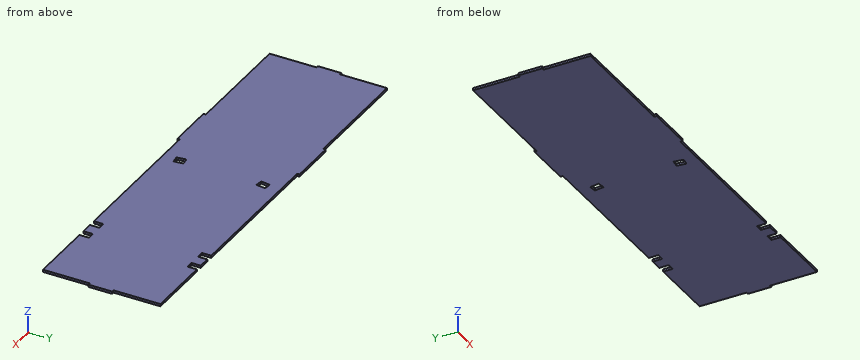
```python
from build123d import *

# Parameters (mm, degrees)
SKETCH_1_W          = 2
SKETCH_1_H          = 20
SKETCH_1_W_2        = 40
SKETCH_1_H_2        = 2
EXTRUDE_1_DEPTH     = 2
CUT_EXTRUDE_1_DEPTH = 10
SKETCH_3_W          = 6
SKETCH_3_H          = 8
CUT_EXTRUDE_2_DEPTH = 2
SKETCH_4_W          = 6
SKETCH_4_H          = 8
CUT_EXTRUDE_3_DEPTH = 2


with BuildPart() as part:
    # 草图1 → 凸台-拉伸1 (new body)
    with BuildSketch(Plane.XY):
        with Locations((1, 50)):
            Rectangle(SKETCH_1_W, SKETCH_1_H)
        Polygon((2, 40), (2, 0), (100, 0), (140, 0), (350, 0), (350, 40), (350, 60), (350, 100), (140, 100), (100, 100), (2, 100), (2, 60), align=None)
        with Locations((120, 101)):
            Rectangle(SKETCH_1_W_2, SKETCH_1_H_2)
        with Locations((120, -1)):
            Rectangle(SKETCH_1_W_2, SKETCH_1_H_2)
        with Locations((351, 50)):
            Rectangle(SKETCH_1_W, SKETCH_1_H)
    extrude(amount=EXTRUDE_1_DEPTH)

    # 草图2 → 切除-拉伸1 (cut)
    with BuildSketch(Plane(origin=(0, 0, 0), x_dir=(-1, 0, 0), z_dir=(0, 0, -1))):
        Polygon((-168.407456688, 81.069541445), (-169.466891791, 88.999080981), (-163.519737138, 89.793657309), (-162.460302035, 81.864117772), align=None)
        Polygon((-162.460302035, 18.135882228), (-168.407456688, 18.930458555), (-169.466891791, 11.000919019), (-163.519737138, 10.206342691), align=None)
    extrude(amount=-CUT_EXTRUDE_1_DEPTH, mode=Mode.SUBTRACT)

    # 草图3 → 切除-拉伸2 (cut)
    with BuildSketch(Plane.XY.offset(2)):
        with Locations((291.061030213, 96)):
            Rectangle(SKETCH_3_W, SKETCH_3_H)
        with Locations((291.061030213, 4)):
            Rectangle(SKETCH_3_W, SKETCH_3_H)
    extrude(amount=-CUT_EXTRUDE_2_DEPTH, mode=Mode.SUBTRACT)

    # 草图4 → 切除-拉伸3 (cut)
    with BuildSketch(Plane.XY.offset(2)):
        with Locations((274.986515691, 4)):
            Rectangle(SKETCH_4_W, SKETCH_4_H)
        with Locations((274.986515691, 96)):
            Rectangle(SKETCH_4_W, SKETCH_4_H)
    extrude(amount=-CUT_EXTRUDE_3_DEPTH, mode=Mode.SUBTRACT)


solid = part.part
```
Here's how the part is built. I have some questions about the finished solid (model axes, mm). Coordinates: 2 decimals unless noted, no trailing zeros. Order: outer loops, then holes, each group sorted by start corner. A loop starts at its lowest first (then second) coordinate and runs counter-clockwise, first axis right, second up. Notation, with made-up numbers: M 9.5,43 L 19.5,43 A28 cw 19.5,67 Z; hole C 64.5,42 d4. An arc over 180 degrees is marked long. Answer as a JSON object with one key per item and string values. Group by question number.
(1) I need wall thicknesses on probe 1 along X at (y, z) = (97.5, 1.15); probe 2 along Y at (x, z) = (189.5, 1.2); probe 3 along X at (y, z) = (70, 1.2). Which ranges of each line are inside material? Lowest first, please.
(2) For pin 1 (1 mm diameter, centred on x = 1, z = 1.5, fed in from +Y); pin 2 (1 mm diameter, centred on x = 81, z = 1, fed in from +Y); pin 3 (1 mm diameter, centred on y = 4.5, z = 1, fed in from -X), each with a flat end and sliding along its axis, tell me the tip position at first contact or that it passes through.
(3) Suppose I cut it at B-B, the plane z = 0.8. State how many separate pieces and enclosed holes the cut face has, then the cut area to 3 significant figures.
(4) Suppose I cut it at C-C, the plane x = 89. Please give me the cut outline in (y, z), then the cut area to 3 significant figures.
(5) Suppose I cut it at A-A, the plane y = 15. Please give me the cut outline in (x, z).
Values found:
{
 "1": {"probe 1": "x = 2 to 271.99, 277.99 to 288.06, 294.06 to 350", "probe 2": "y = 0 to 100", "probe 3": "x = 2 to 350"},
 "2": {"pin 1": "stops at y = 60", "pin 2": "stops at y = 100", "pin 3": "stops at x = 2"},
 "3": {"separate pieces": "1", "enclosed holes": "2", "area": "34,800 mm^2"},
 "4": {"outline": "M 0,0 L 100,0 L 100,2 L 0,2 Z", "area": "200 mm^2"},
 "5": {"outline": "M 2,0 L 162.88,0 L 162.88,2 L 2,2 Z; M 168.93,0 L 350,0 L 350,2 L 168.93,2 Z"}
}
